The drawing under review shows one solid part. Ordinate dimensions are in mm from its lowest x, y, z. Round coordinates to 2 decimals unless told otherwise and drop trailing zeros. Write each loop counter-clockwise with the first axis right and the second up, starting at its lowest first coordinate (ties: lowest second). Pieces come first, ordered by that corner, then holes. Notation, with made-up numbers: M -10,-34 L 7,-34 A24 cw 7,-11 Z; hole C -22.5,34.25 d7. An arc over 180 degrees is marked long. One line per item, written item: value. Start each with the question number.
1) Take a section at B-B, the plane y = 65. Write out the cut boundary in (x, z).
2) Take a section at D-D, the plane z = 23. Write out the cut boundary in (x, y), and give its area (3 significant figures).
3) Wall thickness on probe 1 along X at (y, z) = (65, 17.25); probe 2 along Y at (x, z) = (70, 2.5); probe 3 along Y at (x, z) = (70, 20.5): over which ranges is each line inside the solid? List them lowest first.
4) For P1, Ø8, axis at x = 116.5, y = 75, coming from the +Z side, flat-tipped, find the tip position at first contact; note if it passes through.
5) Take a section at A-A, the plane x = 70. Write out the cut boundary in (y, z), and give its area (3 significant figures).
6) Take a section at C-C, the plane z = 2.5. Write out the cut boundary in (x, y), and give its area (3 significant figures).
7) Mouldability with a two-part tool opening along Y and no side actions: class the marked faces 1, 2 and 3 as +Y half, -Y half, draft (parallel to the pull), parting line (faces both ways), or undercut.
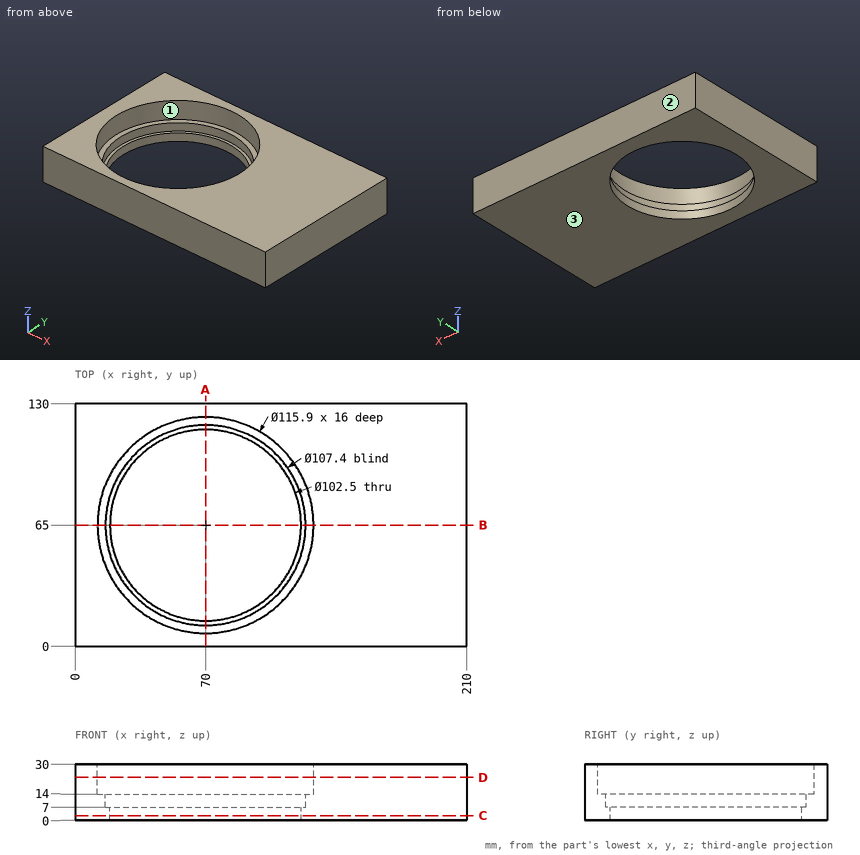
Checked values:
1. outline: M 0,0 L 18.75,0 L 18.75,7 L 16.3,7 L 16.3,14 L 12.05,14 L 12.05,30 L 0,30 Z; M 121.25,0 L 210,0 L 210,30 L 127.95,30 L 127.95,14 L 123.7,14 L 123.7,7 L 121.25,7 Z
2. outline: M 0,0 L 210,0 L 210,130 L 0,130 Z; hole C 70,65 d115.9
2. area: 16,700 mm2
3. probe 1: x = 0 to 12.05, 127.95 to 210
3. probe 2: y = 0 to 13.75, 116.25 to 130
3. probe 3: y = 0 to 7.05, 122.95 to 130
4. P1: stops at z = 7
5. outline: M 0,0 L 13.75,0 L 13.75,7 L 11.3,7 L 11.3,14 L 7.05,14 L 7.05,30 L 0,30 Z; M 116.25,0 L 130,0 L 130,30 L 122.95,30 L 122.95,14 L 118.7,14 L 118.7,7 L 116.25,7 Z
5. area: 576 mm2
6. outline: M 0,0 L 210,0 L 210,130 L 0,130 Z; hole C 70,65 d102.5
6. area: 19,000 mm2
7. face 1: undercut
7. face 2: +Y half
7. face 3: draft
